Geometry check sheet. Reference: drawing and pictorial views, mm from the part's lowest x, y, z. A direction names the side the tool comes from. Coordinates: 2 decimals unless noted, no trailing zeros. Loops run counter-clockwise (first coordinate to the right, second up) from the corner with the lowest first, then second, coordinate; pieces in that order, holes last.
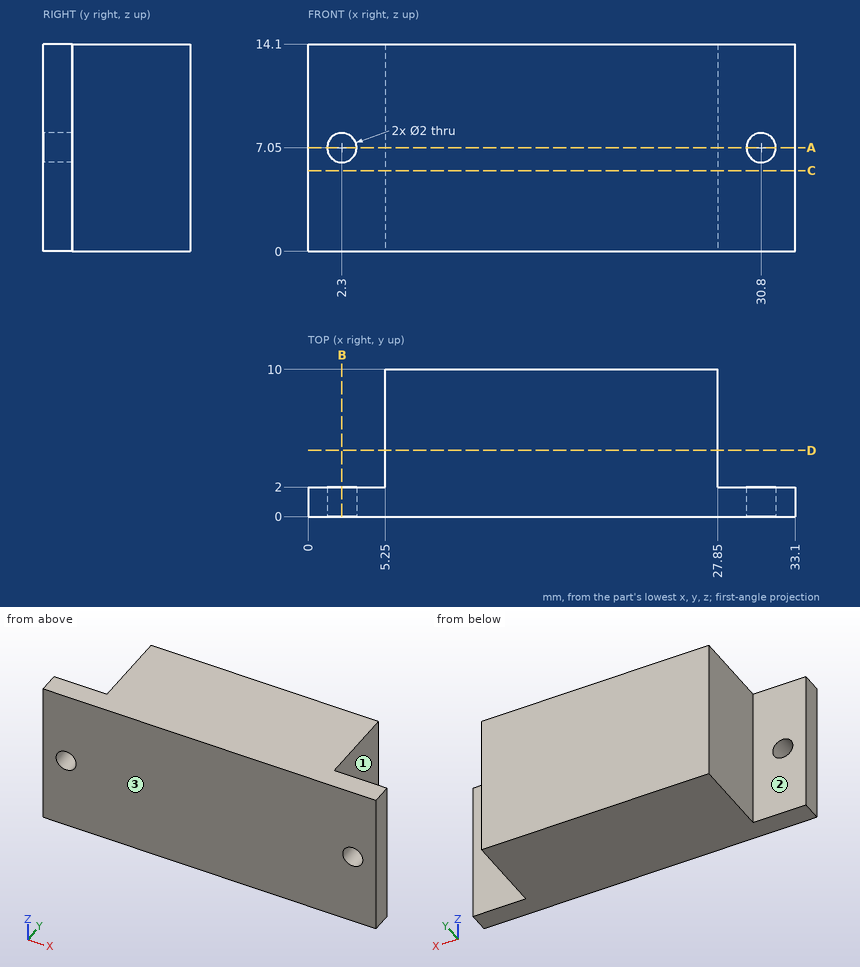
1) Section check B-B on x = 2.3. Record the cut outline in (y, z).
Data:
outline: (0, 0) - (2, 0) - (2, 6.05) - (0, 6.05) - close; (0, 8.05) - (2, 8.05) - (2, 14.1) - (0, 14.1) - close
2) Depth check by flat-ended pin: pin 1 (4 mm diameter, centred on y = 8, z = 6, fed in from +X); pin 2 (1.6 mm diameter, centred on x = 2, z = 4, fed in from +Y); pin 3 (2.5 mm diameter, centred on y = 4, z = 7.5, fed in from -X). Enter the tip coordinate at first touch or a pass-through.
Data:
pin 1: stops at x = 27.85
pin 2: stops at y = 2
pin 3: stops at x = 5.25
3) Section check D-D on y = 4.5. Record the cut outline in (x, z).
Data:
outline: (5.25, 0) - (27.85, 0) - (27.85, 14.1) - (5.25, 14.1) - close
4) Section check C-C on z = 5.5. Record the cut outline in (x, y), and give its area (3 significant figures).
Data:
outline: (0, 0) - (33.1, 0) - (33.1, 2) - (27.85, 2) - (27.85, 10) - (5.25, 10) - (5.25, 2) - (0, 2) - close
area: 247 mm2
5) Material ranges on probe 1 along X at (y, z) = (0.8, 7.05); probe 2 along Z at (x, y) = (30.8, 0.9); probe 3 along X at (y, z) = (9, 12.25), recorded low to high.
Data:
probe 1: x = 0 to 1.3, 3.3 to 29.8, 31.8 to 33.1
probe 2: z = 0 to 6.05, 8.05 to 14.1
probe 3: x = 5.25 to 27.85
6) Section check A-A on z = 7.05. Record the cut outline in (x, y).
Data:
outline: (0, 0) - (1.3, 0) - (1.3, 2) - (0, 2) - close; (3.3, 0) - (29.8, 0) - (29.8, 2) - (27.85, 2) - (27.85, 10) - (5.25, 10) - (5.25, 2) - (3.3, 2) - close; (31.8, 0) - (33.1, 0) - (33.1, 2) - (31.8, 2) - close
7) Access from +Z, -Z, +X, -X, +Y, -Y to the whole of each face (thin tool, end or side, straight path). Record for the marked faces 1, 2 and 3.
Data:
face 1: +Z, -Z, +X, +Y
face 2: +Z, -Z, -X, +Y
face 3: +Z, -Z, +X, -X, -Y
